Could you check a few things on this model? Use its own coordinates, in mm. A direction names the side the tool comes from. Round coordinates to 2 decimals unless told otherwise and drop trailing zeros. Write each loop counter-clockwise with the first axis right and the second up, starting at its lowest first coordinate (ties: lowest second). Pieces come first, ordered by that corner, then holes. Notation, with made-up numbers: (-12, 16) -> (3, 16) arc R8 cw to (3, 22) -> close; hole circle Ø6 at (-0.5, 56). An arc over 180 degrees is marked (long way). Answer in a Markdown table with one row per item.
from build123d import *

# Parameters (mm, degrees)
F0_R     = 32.004
F1_DEPTH = 4.445
F2_R     = 21.971
F3_DEPTH = 15.748
F4_R     = 1.27
F6_DEPTH = 1.27
F8_DEPTH = 0.508


with BuildPart() as f1:
    # F0 (on Top) → F1 (new body)
    with BuildSketch(Plane.XY):
        with Locations((0.0734815403, -0.3912560351)):
            Circle(F0_R)
    extrude(amount=F1_DEPTH)

    # F2 (on face) → F3 (join)
    with BuildSketch(Plane.XY.offset(4.445)):
        Circle(F2_R)
    extrude(amount=F3_DEPTH)

    # F4
    f4_edges = [f1.edges().sort_by_distance(p)[0] for p in [
        (-31.930518, -0.391256, 4.445),
    ]]
    fillet(f4_edges, radius=F4_R)

    # F5 (on face) → F6 (cut)
    with BuildSketch(Plane.XY.offset(20.193)):
        with BuildLine():
            ThreePointArc((11.5169007331, -4.2504528537), (-5.8335664103, -4.8630391768), (-3.625406418, 12.3572396114))
            Line((-3.625406418, 12.3572396114), (-3.625406418, 15.8741623163))
            Line((-3.625406418, 15.8741623163), (-5.2373292856, 14.9949323386))
            Line((-5.2373292856, 14.9949323386), (-9.9754063413, 17.78))
            Line((-9.9754063413, 17.78), (-13.4434830397, 14.9949323386))
            Line((-13.4434830397, 14.9949323386), (-10.3661753237, 10.1591628045))
            Line((-10.3661753237, 10.1591628045), (-12.0757911354, 6.153778173))
            Line((-12.0757911354, 6.153778173), (-17.78, 5.1280092448))
            Line((-17.78, 5.1280092448), (-17.78, 0.4876240855))
            Line((-17.78, 0.4876240855), (-12.1734831482, -1.0266067693))
            Line((-12.1734831482, -1.0266067693), (-10.3661753237, -5.0808377564))
            Line((-10.3661753237, -5.0808377564), (-14.225021936, -9.9654532969))
            Line((-14.225021936, -9.9654532969), (-10.8057912439, -13.4823769331))
            Line((-10.8057912439, -13.4823769331), (-5.6280987337, -9.9166072905))
            Line((-5.6280987337, -9.9166072905), (-1.6227141023, -11.6262231022))
            Line((-1.6227141023, -11.6262231022), (0, -17.78))
            Line((0, -17.78), (4.4342088513, -17.78))
            Line((4.4342088513, -17.78), (5.8995936997, -11.4308381453))
            Line((5.8995936997, -11.4308381453), (10.0026708096, -9.8677603528))
            Line((10.0026708096, -9.8677603528), (14.9849783629, -13.2381459698))
            Line((14.9849783629, -13.2381459698), (17.78, -9.7212223336))
            Line((17.78, -9.7212223336), (11.5169007331, -4.2504528537))
        make_face()
        with BuildLine():
            add(Edge.make_bspline(
                [(7.2628180496, 15.8830489963), (7.764120513, 15.8547054313), (8.7931376229, 15.7965249604), (10.4249300167, 15.2148196487), (11.8099126054, 14.2323930058), (13.1704291206, 12.5947806565), (14.0438131033, 10.7817202185), (14.1201673867, 7.3393260802), (13.7194691328, 5.5139226252), (13.0765966002, 4.3745110609), (12.4961633849, 3.1101795931), (10.8585799754, 2.0034232369), (10.0201954446, 1.6327368317), (8.7603057074, 1.291574238), (8.0080404878, 1.0878700996)],
                knots=[0, 0, 0, 0, 0.0772193353, 0.1585071351, 0.2400871058, 0.3296102404, 0.4189216979, 0.5342087706, 0.6199032215, 0.6892989221, 0.7632939871, 0.8489473746, 0.9098082689, 1, 1, 1, 1], degree=3))
            Line((7.2628180496, 15.8830489963), (-2.8727587778, 15.8830489963))
            Line((-2.8727587778, 15.8830489963), (-2.8727587778, -6.3826409169))
            Line((-2.8727587778, -6.3826409169), (2.9688859358, -6.3826409169))
            Line((2.9688859358, -6.3826409169), (2.9688859358, 1.0878700996))
            Line((2.9688859358, 1.0878700996), (8.0080404878, 1.0878700996))
        make_face()
        with BuildLine():
            Line((2.9969443567, 11.2640913576), (5.9029692784, 11.2640913576))
            add(Edge.make_bspline(
                [(5.9029692784, 11.2640913576), (6.311247704, 11.169172309), (7.117729351, 10.9816765566), (7.8395571972, 9.97335199), (8.1597875123, 9.2817549766), (8.2415328063, 8.4012900963), (8.2114096294, 7.6759192789), (7.7218664719, 6.5872887351), (7.0554159923, 6.0180518678), (6.3806756136, 5.8354795836), (6.0261930339, 5.7395631447)],
                knots=[0, 0, 0, 0, 0.14072062, 0.2779686368, 0.3897367685, 0.5061439342, 0.6157367861, 0.751736381, 0.8695718667, 1, 1, 1, 1], degree=3))
            Line((6.0261930339, 5.7395631447), (2.9969443567, 5.7395631447))
            Line((2.9969443567, 5.7395631447), (2.9969443567, 11.2640913576))
        make_face(mode=Mode.SUBTRACT)
    extrude(amount=-F6_DEPTH, mode=Mode.SUBTRACT)

    # F7 (on face) → F8 (cut)
    with BuildSketch(Plane(origin=(0, 0, 0), x_dir=(1, 0, 0), z_dir=(0, 0, -1))):
        with BuildLine():
            ThreePointArc((11.3601768389, 1.597710303), (20.1967129552, 12.4455869556), (10.6863165274, 22.7078069001))
            Line((10.6863165274, 22.7078069001), (-3.9929486811, 22.7078069001))
            Line((-3.9929486811, 22.7078069001), (-3.9929486811, -9.0245176107))
            Line((-3.9929486811, -9.0245176107), (4.2410902679, -9.0245176107))
            Line((4.2410902679, -9.0245176107), (4.2410902679, 1.597710303))
            Line((4.2410902679, 1.597710303), (11.3601768389, 1.597710303))
        make_face()
        with BuildLine():
            Line((4.2392467149, 16.0716325045), (8.5572467149, 16.0716325045))
            ThreePointArc((8.5572467149, 16.0716325045), (11.67463885, 12.1071133763), (8.5572467149, 8.1425942481))
            Line((8.5572467149, 8.1425942481), (4.2392467149, 8.1425942481))
            Line((4.2392467149, 8.1425942481), (4.2392467149, 16.0716325045))
        make_face(mode=Mode.SUBTRACT)
        with BuildLine():
            ThreePointArc((16.6819114238, -6.0063162819), (-8.4387461135, -7.4533040262), (-5.2131637931, 17.5013914704))
            Line((-5.2131637931, 17.5013914704), (-5.2131637931, 22.5260201842))
            Line((-5.2131637931, 22.5260201842), (-7.6528675854, 21.0447721183))
            Line((-7.6528675854, 21.0447721183), (-14.565362595, 25.4))
            Line((-14.565362595, 25.4), (-19.0091095865, 21.5094778687))
            Line((-19.0091095865, 21.5094778687), (-14.6524952725, 14.190364629))
            Line((-14.6524952725, 14.190364629), (-17.2083750367, 8.4396339953))
            Line((-17.2083750367, 8.4396339953), (-25.4, 7.1616931818))
            Line((-25.4, 7.1616931818), (-25.4, 0.6350930198))
            Line((-25.4, 0.6350930198), (-17.2410104424, -1.336485846))
            Line((-17.2410104424, -1.336485846), (-14.6524952725, -7.1198018268))
            Line((-14.6524952725, -7.1198018268), (-20.1845727861, -14.2024941742))
            Line((-20.1845727861, -14.2024941742), (-15.4662290588, -18.9843121916))
            Line((-15.4662290588, -18.9843121916), (-7.9194987193, -14.0996957198))
            Line((-7.9194987193, -14.0996957198), (-2.2044987418, -16.6396964341))
            Line((-2.2044987418, -16.6396964341), (0, -25.4))
            Line((0, -25.4), (6.3412087038, -25.4))
            Line((6.3412087038, -25.4), (8.3538619801, -16.2688288838))
            Line((8.3538619801, -16.2688288838), (14.0649145469, -14.0794068575))
            Line((14.0649145469, -14.0794068575), (21.5155947953, -18.9242325723))
            Line((21.5155947953, -18.9242325723), (25.1302085817, -13.9663480222))
            Line((25.1302085817, -13.9663480222), (16.6819114238, -6.0063162819))
        make_face()
    extrude(amount=-F8_DEPTH, mode=Mode.SUBTRACT)


solid = f1.part
1) For pin 1 (0.6 mm diameter, centred on y = 15, z = 20, fed in from -X); pin 2 (0.6 mm diameter, centred on x = 0.5, z = 0, fed in from -Y) (3 decimals); pin 3 (0.6 mm diameter, centred on x = 0, z = 19.5, fed in from -Y); pin 4 (5 mm diameter, centred on x = -13, y = -6.5, fed in from -Z), each with a flat end and sliding along its axis, tell me the tip position at first contact or that it passes through.
Findings:
| item | result |
|---|---|
| pin 1 | stops at x = -16.33 |
| pin 2 | stops at y = -32.395 |
| pin 3 | stops at y = -21.97 |
| pin 4 | stops at z = 0 |
2) Thinking about a two-plate mould opening in Y: for faces 1 (the face through (-11.21, 8.18, 19.57)), 2 (the face through (20.956, 6.599, 12.209)), 3 (the face through (8, -12, 0)), which applies, +Y half, -Y half, draft (parallel to the pull), parting line (faces both ways), or undercut?
Findings:
| item | result |
|---|---|
| face 1 | undercut |
| face 2 | parting line |
| face 3 | draft |
3) For faces 4 (the face through (6, 9, 20.193)), 5 (the face through (-0.823, -14.66, 19.567)), 6 (the face through (-8, 9, 0.508)), which set-ups out of +Z, -Z, +X, -X, +Y, -Y let a thin tool reach every point of the face, with its end or its side?
Findings:
| item | result |
|---|---|
| face 4 | +Z, +X, -X, +Y, -Y |
| face 5 | +Z |
| face 6 | -Z |
4) Please list where these lines run through material, in increasing order: line 1 (Z direction, x = -4, y = 28.5) (3 decimals); line 2 (X direction, y = -0.5, z = 12.75); line 3 (Z direction, x = 0.5, y = 16.5).
Findings:
| item | result |
|---|---|
| line 1 | z = 0 to 4.445 |
| line 2 | x = -21.97 to 21.97 |
| line 3 | z = 0.51 to 20.19 |
5) Imagine slicing it at A-A, the plane z = 5.75. Please give me the cut outline in (x, y).
Findings:
| item | result |
|---|---|
| outline | circle Ø43.94 at (0, 0) |
